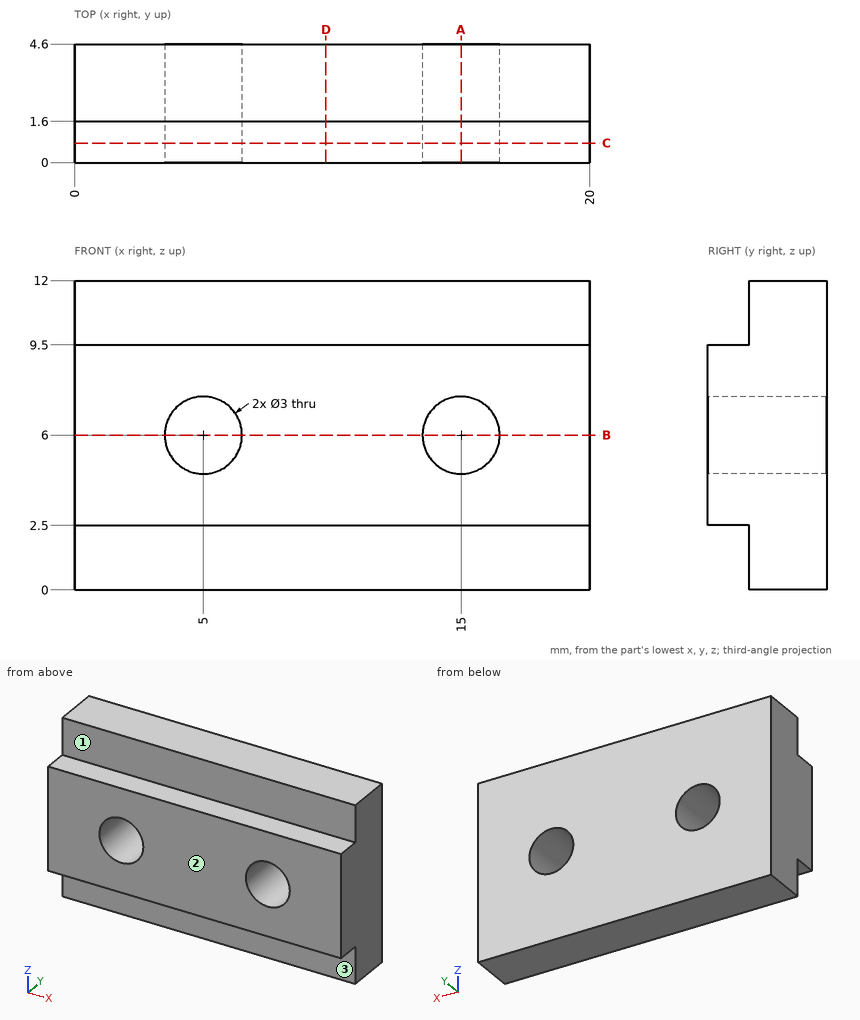
Geometry: see drawing. Coordinates: mm, zero at the bounding-box minimum. A direction names the side the tool comes from. Coordinates: 2 decimals unless noted, no trailing zeros. Write each loop counter-clockwise with the first axis right and the second up, starting at its lowest first coordinate (ties: lowest second). Pieces come first, ordered by that corner, then holes. Notation, with made-up numbers: M 18,-32 L 24,-32 A27 cw 24,3 Z; hole C 6.25,-13.75 d9. An arc over 180 degrees is marked long. Use CSV: the item, a comma, the result in double quotes. Start each with the question number.
1. Ray query, probe 1 along Z at (x, y) = (15, 2.6); probe 2 along X at (y, z) = (1.85, 7); probe 3 along X at (y, z) = (0.5, 7.25). Return the intervals inside material, ascending.
2. Cut plane A-A on x = 15. Return the cut outline in (y, z).
3. Cut plane D-D on x = 9.75. Return the cut outline in (y, z), plus the area to 3 significant figures.
4. Cut plane B-B on z = 6. Return the cut outline in (x, y).
5. Cut plane C-C on y = 0.75. Return the cut outline in (x, z).
6. First-contact query: P1, Ø5, axis at x = 15, z = 6, coming from the +Y side; P2, Ø1.3, axis at x = 15, y = 0.5, coming from the +Z side; P3, Ø0.5, axis at x = 10.5, y = 1, coming from the -Z side; P4, Ø1.2, axis at x = 6, z = 11, coming from the -Y side. Flat tips, straight axial feed; report the tip coordinate or a pass-through.
7. Reachability of the marked faces 1, 2 and 3 from +Z, -Z, +X, -X, +Y, -Y: full face, straight path, thin tool, end or side. Return the list, or none.
Entries:
1,probe 1,"0 to 4.5, 7.5 to 12"
1,probe 2,"0 to 3.88, 6.12 to 13.88, 16.12 to 20"
1,probe 3,"0 to 4.17, 5.83 to 14.17, 15.83 to 20"
2,outline,"M 0,2.5 L 1.6,2.5 L 1.6,0 L 4.6,0 L 4.6,4.5 L 0,4.5 Z; M 0,7.5 L 4.6,7.5 L 4.6,12 L 1.6,12 L 1.6,9.5 L 0,9.5 Z"
3,outline,"M 0,2.5 L 1.6,2.5 L 1.6,0 L 4.6,0 L 4.6,12 L 1.6,12 L 1.6,9.5 L 0,9.5 Z"
3,area,"47.2 mm²"
4,outline,"M 0,0 L 3.5,0 L 3.5,4.6 L 0,4.6 Z; M 6.5,0 L 13.5,0 L 13.5,4.6 L 6.5,4.6 Z; M 16.5,0 L 20,0 L 20,4.6 L 16.5,4.6 Z"
5,outline,"M 0,2.5 L 20,2.5 L 20,9.5 L 0,9.5 Z; hole C 5,6 d3; hole C 15,6 d3"
6,P1,"y = 4.6"
6,P2,"z = 9.5"
6,P3,"z = 2.5"
6,P4,"y = 1.6"
7,face 1,"+Z, +X, -X, -Y"
7,face 2,"+Z, -Z, +X, -X, -Y"
7,face 3,"-Z, +X, -X, -Y"
